Work out the finished part from the listing and answer in its coordinate system (mm). A direction names the side the tool comes from. Round coordinates to 2 decimals unless told otherwise and drop trailing zeros. Order: outer loops, then holes, each group sorted by start corner. A loop starts at its lowest first (then second) coordinate and runs counter-clockwise, first axis right, second up. Notation, with made-up numbers: M 30,39 L 87,39 A23 ccw 87,55 Z; hole C 67.25,10.5 d1. An arc over 180 degrees is marked long. Return JSON: item names as keys, results as strings.
from build123d import *

# Parameters (mm, degrees)
SKETCH1_R           = 9.5025
SKETCH1_W           = 88.9
SKETCH1_H           = 3
BOSS_EXTRUDE1_DEPTH = 3
CUT_EXTRUDE1_DEPTH  = 4
CUT_EXTRUDE2_DEPTH  = 127
FILLET1_R           = 3.81
FILLET2_R           = 1.27
FILLET3_R           = 5.08
SKETCH4_R           = 3.5025
CUT_EXTRUDE3_DEPTH  = 16.002


with BuildPart() as part:
    # Sketch1 → Boss-Extrude1 (new body)
    with BuildSketch(Plane.XY):
        with BuildLine():
            Line((-11.934096284, 4.34365582), (14.127838637, 75.948233524))
            ThreePointArc((14.127838637, 75.948233524), (18.77751418, 82.007808666), (26.061934921, 84.304577704))
            Line((26.061934921, 84.304577704), (152.474181009, 84.304577704))
            Line((152.474181009, 84.304577704), (152.474181009, 58.904577704))
            Line((152.474181009, 58.904577704), (66.968059304, 58.904577704))
            ThreePointArc((66.968059304, 58.904577704), (40.744144634, 50.636209169), (24.005312681, 28.821738657))
            Line((24.005312681, 28.821738657), (11.934096284, -4.34365582))
            ThreePointArc((11.934096284, -4.34365582), (-4.34365582, -11.934096284), (-11.934096284, 4.34365582))
        make_face()
        Circle(SKETCH1_R, mode=Mode.SUBTRACT)
        with Locations((100.404181009, 76.804577704)):
            Rectangle(SKETCH1_W, SKETCH1_H, mode=Mode.SUBTRACT)
    extrude(amount=BOSS_EXTRUDE1_DEPTH)

    # Sketch2 → Cut-Extrude1 (cut, through all)
    with BuildSketch(Plane.XY.offset(3)):
        Polygon((27.008098555, 61.075884743), (9.633475274, 13.339499607), (4.26622335, 24.849608502), (21.640846631, 72.585993638), align=None)
    extrude(amount=-CUT_EXTRUDE1_DEPTH, mode=Mode.SUBTRACT)

    # Sketch3 → Cut-Extrude2 (cut)
    with BuildSketch(Plane.XY.offset(3)):
        Polygon((30.777663682, 71.512392484), (28.523924397, 53.747624001), (54.773358423, 71.512392484), align=None)
        Polygon((64.436448885, 65.362999195), (69.566826389, 73.272331181), (120.366826389, 73.272331181), (115.236448885, 65.362999195), align=None)
    extrude(amount=-CUT_EXTRUDE2_DEPTH, mode=Mode.SUBTRACT)

    # Fillet1
    fillet1_edges = [part.edges().sort_by_distance(p)[0] for p in [
        (27.008098555, 61.075884743, 1.5),
        (4.26622335, 24.849608502, 1.5),
        (30.777663682, 71.512392484, 1.5),
        (115.236448885, 65.362999195, 1.5),
        (69.566826389, 73.272331181, 1.5),
    ]]
    fillet(fillet1_edges, radius=FILLET1_R)

    # Fillet2
    fillet2_edges = [part.edges().sort_by_distance(p)[0] for p in [
        (9.633475274, 13.339499607, 1.5),
        (21.640846631, 72.585993638, 1.5),
        (54.773358423, 71.512392484, 1.5),
        (28.523924397, 53.747624001, 1.5),
        (64.436448885, 65.362999195, 1.5),
        (120.366826389, 73.272331181, 1.5),
    ]]
    fillet(fillet2_edges, radius=FILLET2_R)

    # Fillet3
    fillet3_edges = [part.edges().sort_by_distance(p)[0] for p in [
        (152.474181009, 84.304577704, 1.5),
        (152.474181009, 58.904577704, 1.5),
    ]]
    fillet(fillet3_edges, radius=FILLET3_R)

    # Sketch4 → Cut-Extrude3 (cut)
    with BuildSketch(Plane.XY.offset(3)):
        with Locations((141.694177318, 66.514238531)):
            Circle(SKETCH4_R)
        with Locations((129.235425653, 66.514238531)):
            Circle(SKETCH4_R)
    extrude(amount=-CUT_EXTRUDE3_DEPTH, mode=Mode.SUBTRACT)


solid = part.part
Item 1: Find section C-C (x = 0). Determine the outline of the cut face in (y, z).
Output:
{"outline": "M -12.7,0 L -9.5,0 L -9.5,3 L -12.7,3 Z; M 9.5,0 L 37.13,0 L 37.13,3 L 9.5,3 Z"}
Item 2: Consider line 1 along Y through (x, z) = (80, 1.2); line 2 along Y through (x, z) = (114.5, 1); line 3 along X through (y, z) = (76, 0.5). Determine where each line is inside the solid, lowest interval first. Write a range as [from, to].
Output:
{"line 1": "y = [58.9, 65.36], [73.27, 75.3], [78.3, 84.3]", "line 2": "y = [58.9, 65.6], [73.27, 75.3], [78.3, 84.3]", "line 3": "x = [14.15, 55.95], [144.85, 152.47]"}
Item 3: Which of the six approach directions +Z, -Z, +X, -X, +Y, -Y give full straight-line access (tool end or side, diameter ignored) to faces 1 (the cylindrical face through (150.9, 82.9, 1.5)), 2 (the flat face through (18.686, 38.21, 1.521))?
Output:
{"face 1": "+Z, -Z, +X, +Y", "face 2": "+Z, -Z"}
Item 4: Find section A-A (x = 110). Determine the outline of the cut face in (y, z).
Output:
{"outline": "M 58.9,0 L 65.36,0 L 65.36,3 L 58.9,3 Z; M 73.27,0 L 75.3,0 L 75.3,3 L 73.27,3 Z; M 78.3,0 L 84.3,0 L 84.3,3 L 78.3,3 Z"}
Item 5: Find section D-D (z = 0.95). State how many separate pieces and enclosed holes the cut face has, plus the area to 3 significant figures.
Output:
{"separate pieces": "1", "enclosed holes": "7", "area": "3,880 mm^2"}
Item 6: The mould has two halves that part along X. Classify faces 3 (the flat face through (52, 61, 3)), 4 (the cylindrical face through (18.689, 81.945, 1.479)), 5 (the flat face through (24.615, 66.208, 1.521)): pulls with the +X half, pulls with the -X half, needs draft (parallel to the pull), parting line crosses it, or undercut.
Output:
{"face 3": "needs draft", "face 4": "pulls with the -X half", "face 5": "undercut"}
Item 7: Find section B-B (y = 40). Determine the outline of the cut face in (x, z).
Output:
{"outline": "M 1.04,0 L 9.78,0 L 9.78,3 L 1.04,3 Z; M 19.34,0 L 29.94,0 L 29.94,3 L 19.34,3 Z"}
Item 8: Each of these flat-tipped pins is pushed along its axis until it touches: pin 1 (1.5 mm diameter, centred on y = 35.5, z = 0.5, fed in from +X); pin 2 (0.9 mm diameter, centred on x = 106.5, z = 1.5, fed in from -Y). Where does it stop, or does it pass through?
Output:
{"pin 1": "stops at x = 27.49", "pin 2": "stops at y = 58.9"}
